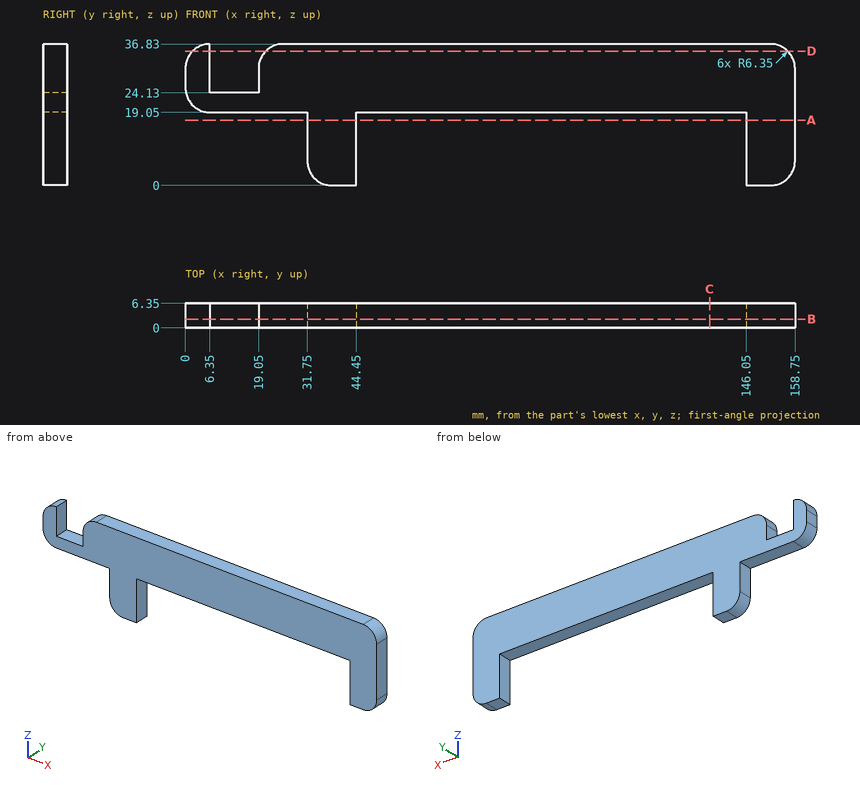
Answer from the drawing. Dimensions are ordinates in mm from the lowest x, y and z of the part. Give positions to 0.01 mm unless a question says otherwise; leave off trailing zeros. Loops run counter-clockwise (first coordinate to the right, second up) from the corner with the lowest first, then second, coordinate; pieces in that order, holes last. Notation, with made-up numbers: M 34,-3 L 71,-3 A23 ccw 71,27 Z; hole C 52,35.5 d10. An arc over 180 degrees is marked long. One line per item, written item: value.
Q1. A cutting plane is placed at B-B on y = 2.25. Determine the outline of the cut face in (x, z), then the cut area to 3 significant figures.
Working result:
outline: M 0,25.4 A6.35 ccw 6.35,19.05 L 31.75,19.05 L 31.75,6.35 A6.35 ccw 38.1,0 L 44.45,0 L 44.45,19.05 L 146.05,19.05 L 146.05,0 L 152.4,0 A6.35 ccw 158.75,6.35 L 158.75,30.48 A6.35 ccw 152.4,36.83 L 25.4,36.83 A6.35 ccw 19.05,30.48 L 19.05,24.13 L 6.35,24.13 L 6.35,36.83 A6.35 ccw 0,30.48 Z
area: 3,090 mm^2
Q2. A cutting plane is placed at D-D on z = 35. Determine the outline of the cut face in (x, y).
Working result:
outline: M 1.89,0 L 6.35,0 L 6.35,6.35 L 1.89,6.35 Z; M 20.94,0 L 156.86,0 L 156.86,6.35 L 20.94,6.35 Z
Q3. Flat-ended cylindrical pins translate along their axes: P1, Ø3, axis at y = 4, z = 15, coming from the -X side; P2, Ø1.9, axis at x = 25, y = 3, coming from the -Z side; P3, Ø1.9, axis at x = 12.5, y = 3, coming from the +Z side. Find the tip coordinate at first contact, or state that the pin passes through.
Working result:
P1: stops at x = 31.75
P2: stops at z = 19.05
P3: stops at z = 24.13
Q4. A cutting plane is placed at C-C on x = 136.5. Determine the outline of the cut face in (y, z).
Working result:
outline: M 0,19.05 L 6.35,19.05 L 6.35,36.83 L 0,36.83 Z
Q5. Find the intervals of material crossed by line 1 (X direction, y = 5.25, z = 14.5); line 2 (X direction, y = 5, z = 29.5); line 3 (Z direction, x = 122, y = 1.5), in increasing order. Write a range as from..to.
Working result:
line 1: x = 31.75..44.45, 146.05..158.75
line 2: x = 0..6.35, 19.05..158.75
line 3: z = 19.05..36.83
Q6. A cutting plane is placed at A-A on z = 17. Determine the outline of the cut face in (x, y).
Working result:
outline: M 31.75,0 L 44.45,0 L 44.45,6.35 L 31.75,6.35 Z; M 146.05,0 L 158.75,0 L 158.75,6.35 L 146.05,6.35 Z
